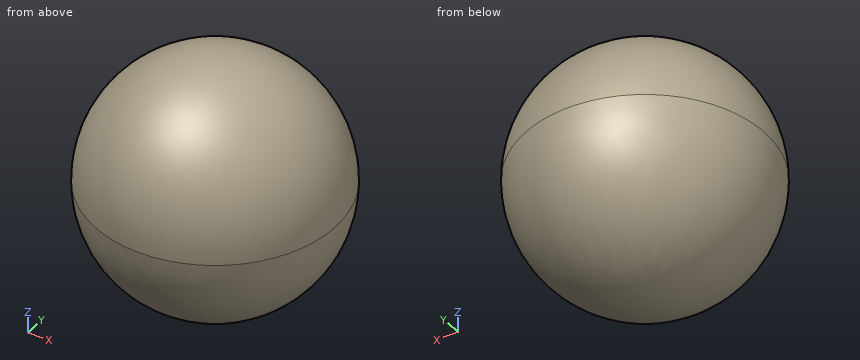
```python
from build123d import *

# Parameters (mm, degrees)
F0_R     = 50.8
F1_DEPTH = 50.8
F2_R     = 50.8
F3_R     = 50.79999


# Not quite as in the source:
# - a fillet or chamfer is up to 0.001 mm smaller than in the source, because OpenCascade refuses the exact size


with BuildPart() as f1:
    # F0 (on Top) → F1 (new body, symmetric)
    with BuildSketch(Plane.XY):
        Circle(F0_R)
    extrude(amount=F1_DEPTH, both=True)

    # F2
    f2_edges = [f1.edges().sort_by_distance(p)[0] for p in [
        (-50.8, 0, 50.8),
    ]]
    fillet(f2_edges, radius=F2_R)

    # F3 (radius 50.8 in the source; OpenCascade refuses exactly that, so slightly less here)
    f3_edges = [f1.edges().sort_by_distance(p)[0] for p in [
        (-50.8, 0, -50.8),
    ]]
    fillet(f3_edges, radius=F3_R)


solid = f1.part
```
Build history of the part. All positions in model axes, mm. Give positions to 0.01 mm unless a question says otherwise; leave off trailing zeros. Loops run counter-clockwise (first coordinate to the right, second up) from the corner with the lowest first, then second, coordinate; pieces in that order, holes last.
Item 1: Slice it at A-A, the plane z = 37.5. List the corners of the cut face in (x, y).
Answers follow:
outline: circle Ø68.54 at (0, 0)
Item 2: Drill centre lines: line 1 (X direction, y = 22, z = 40.5); line 2 (Z direction, x = -2, y = -2); line 3 (Y direction, x = -25, z = 7). Where is each one in solid material? Low to high.
Answers follow:
line 1: x = -21.36 to 21.36
line 2: z = -50.72 to 50.72
line 3: y = -43.67 to 43.67
Item 3: Flat gauge pins, fed straight in: pin 1 (8 mm diameter, centred on y = -20, z = -7.5, fed in from +X); pin 2 (5 mm diameter, centred on x = -19, y = -32, fed in from +Z); pin 3 (2 mm diameter, centred on x = 17, z = -17, fed in from -Y). Where does each tip first touch, or does it go through?
Answers follow:
pin 1: stops at x = 47.74
pin 2: stops at z = 37.09
pin 3: stops at y = -45.27
